For this review, take the finished solid that the model builds, in its own axes (mm). A direction names the side the tool comes from. Give positions to 0.01 mm unless a question says otherwise; leave off trailing zeros. Order: outer loops, then holes, each group sorted by start corner. A loop starts at its lowest first (then second) coordinate and runs counter-clockwise, first axis right, second up. Notation, with made-up numbers: (-17.5, -8) -> (6.5, -8) arc R32 ccw to (6.5, 24) -> close; hole circle Ø5 at (60.5, 53). An arc over 180 degrees is marked (long way). Use CSV: the item, a comma, the result in double quotes. Start each with the question number.
```python
from build123d import *

# Parameters (mm, degrees)
SKETCH_1_W         = 49
SKETCH_1_H         = 23.5
SKETCH_1_R         = 1.5
EXTRUDE_512_DEPTH  = 1
SKETCH_2_R         = 4
EXTRUDE_1244_DEPTH = 10.5
SKETCH_2_3_W       = 9.5
SKETCH_2_3_H       = 5
EXTRUDE_1289_DEPTH = 11.5
SKETCH_2_5_W       = 12
SKETCH_2_5_H       = 12
EXTRUDE_1429_DEPTH = 8.5
SKETCH_2_6_W       = 13
SKETCH_2_6_H       = 10
EXTRUDE_1653_DEPTH = 4.5


with BuildPart() as part:
    # Sketch 1 → Extrude 512 (new body)
    with BuildSketch(Plane.XY):
        Rectangle(SKETCH_1_W, SKETCH_1_H)
        with Locations((-16.5, 8.25)):
            Circle(SKETCH_1_R, mode=Mode.SUBTRACT)
        with Locations((16.5, -8.25)):
            Circle(SKETCH_1_R, mode=Mode.SUBTRACT)
    extrude(amount=EXTRUDE_512_DEPTH)

    # Sketch 2 → Extrude 1244 (add)
    with BuildSketch(Plane.XY.offset(1)):
        with Locations(Location((-20.5, 1.25, 0), (0, 0, 180))):
            Circle(SKETCH_2_R)
        with Locations((20.5, -0.75)):
            Circle(SKETCH_2_R)
    extrude(amount=EXTRUDE_1244_DEPTH)

    # Sketch 2_3 → Extrude 1289 (add)
    with BuildSketch(Plane.XY.offset(1)):
        with Locations((8.75, -9.15)):
            Rectangle(SKETCH_2_3_W, SKETCH_2_3_H)
    extrude(amount=EXTRUDE_1289_DEPTH)

    # Sketch 2_5 → Extrude 1429 (add)
    with BuildSketch(Plane.XY.offset(1)):
        with Locations((-6.5, 5.65)):
            Rectangle(SKETCH_2_5_W, SKETCH_2_5_H)
        with Locations((8, -0.25)):
            Rectangle(SKETCH_2_5_W, SKETCH_2_5_H)
    extrude(amount=EXTRUDE_1429_DEPTH)

    # Sketch 2_6 → Extrude 1653 (add)
    with BuildSketch(Plane.XY.offset(1)):
        with Locations((-5.5, -6.65)):
            Rectangle(SKETCH_2_6_W, SKETCH_2_6_H)
    extrude(amount=EXTRUDE_1653_DEPTH)


solid = part.part
```
1. For faces 1 (the face through (8, -6.25, 5)), 2 (the face through (-6, -11.65, 3)), 3 (the face through (8, 0, 9.5)), 4 (the face through (-7, -0.35, 5)), 5 (the face through (-12.5, 6, 5)), list the 3-axis set-ups (+Z, -Z, +X, -X, +Y, -Y) from which the entire face can be reached by the end or side of a thin tool; tool diameter is ignored.
2. Consider section C-C (z = 9). State the section outline as (x, y) points, plus the area to 3 significant figures.
3. Clearance check with flat-ended pins moving along their axes: P1, Ø4, axis at y = 4, z = 4.5, coming from the -X side; P2, Ø2.5, axis at y = -10, z = 8.5, coming from the -X side; P3, Ø1.3, axis at x = -5.5, z = 2.5, coming from the +Y side. State where each tip first meets the part, or that it passes through.
4. Consider section B-B (z = 2.25). State the section outline as (x, y) points.
5. Draft analysis for pull direction Y (two halves, no side actions). For faces 6 (the face through (-6, -1.65, 3)), 7 (the face through (8, 5.75, 5)), 8 (the face through (-17.326, 3.684, 6.176)), 9 (the face through (2, 0, 5)), state which applies: +Y half, -Y half, draft (parallel to the pull), parting line (faces both ways), or undercut.
6. Consider section A-A (y = 8.25). State the section outline as (x, z) points.
7. Consider section D-D (x = 0.5). State the section outline as (y, z) points, plus the area to 3 significant figures.
8. To check wall thickness, follow L1, parallel to Y at x = -16.5, z = 0.3; L2, parallel to Y at x = 16.5, z = 0.55; L3, parallel to X at y = 0.5, z = 9.25. State the ranges of each line that lie inside material, in increasing order. Write a range as [from, to].
Answer list:
1,face 1,"+Z, +X"
1,face 2,"+Z, +X, -X, -Y"
1,face 3,"+Z, +Y"
1,face 4,"+Z"
1,face 5,"+Z, +Y, -Y"
2,outline,"circle Ø8 at (-20.5, 1.25); (-12.5, -0.35) -> (-0.5, -0.35) -> (-0.5, 11.65) -> (-12.5, 11.65) -> close; (2, -6.25) -> (14, -6.25) -> (14, 5.75) -> (2, 5.75) -> close; (4, -11.65) -> (13.5, -11.65) -> (13.5, -6.65) -> (4, -6.65) -> close; circle Ø8 at (20.5, -0.75)"
2,area,"436 mm2"
3,P1,"x = -24.43"
3,P2,"x = 4"
3,P3,"y = 11.65"
4,outline,"circle Ø8 at (-20.5, 1.25); (-12.5, -0.35) -> (-0.5, -0.35) -> (-0.5, 11.65) -> (-12.5, 11.65) -> close; (-12, -11.65) -> (1, -11.65) -> (1, -1.65) -> (-12, -1.65) -> close; (2, -6.25) -> (14, -6.25) -> (14, 5.75) -> (2, 5.75) -> close; (4, -11.65) -> (13.5, -11.65) -> (13.5, -6.65) -> (4, -6.65) -> close; circle Ø8 at (20.5, -0.75)"
5,face 6,"undercut"
5,face 7,"+Y half"
5,face 8,"parting line"
5,face 9,"draft"
6,outline,"(-24.5, 0) -> (-18, 0) -> (-18, 1) -> (-24.5, 1) -> close; (-15, 0) -> (24.5, 0) -> (24.5, 1) -> (-0.5, 1) -> (-0.5, 9.5) -> (-12.5, 9.5) -> (-12.5, 1) -> (-15, 1) -> close"
7,outline,"(-11.75, 0) -> (11.75, 0) -> (11.75, 1) -> (-1.65, 1) -> (-1.65, 5.5) -> (-11.65, 5.5) -> (-11.65, 1) -> (-11.75, 1) -> close"
7,area,"68.5 mm2"
8,L1,"[-11.75, 6.75], [9.75, 11.75]"
8,L2,"[-11.75, -9.75], [-6.75, 11.75]"
8,L3,"[-24.43, -16.57], [-12.5, -0.5], [2, 14], [16.7, 24.3]"
